from build123d import *

# Parameters (mm, degrees)
SKETCH_1_W          = 28
SKETCH_1_H          = 33
EXTRUDE_1_DEPTH     = 15
SKETCH_2_R          = 3
CUT_EXTRUDE_1_DEPTH = 5
SKETCH_3_R          = 3
CUT_EXTRUDE_2_DEPTH = 5


with BuildPart() as part:
    # 草图1 → 凸台-拉伸1 (new body)
    with BuildSketch(Plane(origin=(0, 0, 0), x_dir=(1, 0, 0), z_dir=(0, 1, 0))):
        with Locations((14, -16.5)):
            Rectangle(SKETCH_1_W, SKETCH_1_H)
    extrude(amount=EXTRUDE_1_DEPTH)

    # 草图2 → 切除-拉伸1 (cut)
    with BuildSketch(Plane.XY.offset(33)):
        with Locations((15.25, 7.5)):
            Circle(SKETCH_2_R)
    extrude(amount=-CUT_EXTRUDE_1_DEPTH, mode=Mode.SUBTRACT)

    # 草图3 → 切除-拉伸2 (cut)
    with BuildSketch(Plane(origin=(28, 0, 0), x_dir=(0, 0, -1), z_dir=(1, 0, 0))):
        with Locations((-17.75, 7.5)):
            Circle(SKETCH_3_R)
    extrude(amount=-CUT_EXTRUDE_2_DEPTH, mode=Mode.SUBTRACT)


solid = part.part
Can you work these out from the model? Positions are in its coordinate system, mm. A direction names the side the tool comes from. Coordinates: 2 decimals unless noted, no trailing zeros. Order: outer loops, then holes, each group sorted by start corner. A loop starts at its lowest first (then second) coordinate and runs counter-clockwise, first axis right, second up. Notation, with made-up numbers: (51, 15) - (100, 15) arc R11 ccw to (100, 29) - close; hole circle Ø9 at (-19, 5). An arc over 180 degrees is marked (long way). Answer as a JSON object with one key per item and string values. Group by question number.
Q1. We'd pull the mould along Z, two halves only. Please class faces 4 (the face through (14, 0, 16)), 5 (the face through (14, 7, 0)), 6 (the face through (25.535, 7.632, 20.747)): +Z half, -Z half, draft (parallel to the pull), parting line (faces both ways), or undercut.
Q2. On a 3-axis mill with a long thin cutter (end or side, diameter ignored), from which of +Z, -Z, +X, -X, +Y, -Y can I reach the whole of each face in a straight line? I mean faces 1 (the face through (23, 8, 18)), 2 (the face through (14, 15, 16)), 3 (the face through (12.253, 7.632, 30.535)). Say none if no direction works.
Q3. I need wall thicknesses on line 1 (Y direction, x = 24.3, z = 17.75); line 2 (Y direction, x = 25.75, z = 17); line 3 (Z direction, x = 25.75, y = 8.75). Which ranges of each line are inside material? Lowest first, please. Write a range as from..to.
Q4. Imagine slicing it at C-C (z = 17.75). Please give me the cut outline in (x, y).
Q5. Imagine slicing it at D-D (x = 25.5). Please give me the cut outline in (y, z), and give its area (3 significant figures).
Q6. Imagine slicing it at A-A (y = 7.5). Please give me the cut outline in (x, z), and give its area (3 significant figures).
Q7. Will this pin go through, and if not, where does the flat tip stop? P1, Ø1.8, axis at x = 15.5, y = 7, coming from the +Z side.
Q8. Imagine slicing it at B-B (x = 15.25). Please give me the cut outline in (y, z), and give its area (3 significant figures).
Determined:
{
 "1": {"face 4": "draft", "face 5": "-Z half", "face 6": "undercut"},
 "2": {"face 1": "+X", "face 2": "+Z, -Z, +X, -X, +Y", "face 3": "+Z"},
 "3": {"line 1": "y = 0..4.5, 10.5..15", "line 2": "y = 0..4.6, 10.4..15", "line 3": "z = 0..15.02, 20.48..33"},
 "4": {"outline": "(0, 0) - (28, 0) - (28, 4.5) - (23, 4.5) - (23, 10.5) - (28, 10.5) - (28, 15) - (0, 15) - close"},
 "5": {"outline": "(0, 0) - (15, 0) - (15, 33) - (0, 33) - close; hole circle Ø6 at (7.5, 17.75)", "area": "467 mm2"},
 "6": {"outline": "(0, 0) - (28, 0) - (28, 14.75) - (23, 14.75) - (23, 20.75) - (28, 20.75) - (28, 33) - (18.25, 33) - (18.25, 28) - (12.25, 28) - (12.25, 33) - (0, 33) - close", "area": "864 mm2"},
 "7": {"P1": "stops at z = 28"},
 "8": {"outline": "(0, 0) - (15, 0) - (15, 33) - (10.5, 33) - (10.5, 28) - (4.5, 28) - (4.5, 33) - (0, 33) - close", "area": "465 mm2"}
}
